Geometry check sheet. Reference: the model listing, model coordinates, mm. Coordinates: 2 decimals unless noted, no trailing zeros. Write each loop counter-clockwise with the first axis right and the second up, starting at its lowest first coordinate (ties: lowest second). Pieces come first, ordered by that corner, then holes. Notation, with made-up numbers: (-38.5, 12) -> (-29.5, 12) arc R10 cw to (-29.5, 18) -> close; hole circle Ø11 at (28.25, 72). An arc over 180 degrees is marked (long way). Answer as CSV lines item,"result".
Autodesk Inventor part; units mm, degrees
ref_plane "YZ Plane" through (0, 0, 0) normal (1, 0, 0) x (0, 1, 0)
ref_plane "XZ Plane" through (0, 0, 0) normal (0, 1, 0) x (-1, 0, 0)
ref_plane "XY Plane" through (0, 0, 0) normal (0, 0, 1) x (1, 0, 0)
sketch "스케치1" plane through (0, 0, 0) normal (0, 1, 0) x (-1, 0, 0)
  line L0 (195, 76.5) -> (-195, 76.5)
  line L1 (-195, 76.5) -> (-195, -76.5)
  line L2 (-195, -76.5) -> (195, -76.5)
  line L3 (195, -76.5) -> (195, 76.5)
  line L4 (195, 76.5) -> (-195, -76.5) construction
  line L5 (-195, 76.5) -> (195, -76.5) construction
  point P0 (0, 0)
  dimension "d0" = 390
  dimension "d1" = 153
extrude "돌출1" add sketch "스케치1" along normal blind 3
sketch "스케치2" plane through (0, 3, 0) normal (0, 1, 0) x (1, 0, 0)
  line L0 (-101, -167.7961) -> (-101, 220.4195)
  line L1 (-195, 76.5) -> (-195, -76.5)
  line L2 (-195, -76.5) -> (195, -76.5)
  circle A0 centre (-101, -31.5) radius 2
  circle A1 centre (-101, 33.5) radius 2
  line L3 (195, -76.5) -> (195, 76.5)
  line L4 (-91, -255.1075) -> (-91, 213.2428)
  line L5 (-111, -276.0921) -> (-111, 192.2583)
  line L6 (-190, -202.8267) -> (-190, 265.5236)
  line L7 (190, -180.3404) -> (190, 288.01)
  line L8 (-211.2868, -71.5) -> (199.2371, -71.5)
  circle A2 centre (12.5, -49.5) radius 2
  circle A3 centre (77.5, -49.5) radius 2
  circle A4 centre (12.5, 49.5) radius 2
  circle A5 centre (77.5, 49.5) radius 2
  line L9 (12.5, -49.5) -> (99.2818, -49.5) construction
  line L10 (12.5, 49.5) -> (77.5, 49.5) construction
  line L11 (195, 76.5) -> (-195, 76.5)
  dimension "d4" = 94
  dimension "d10" = 4
  dimension "d11" = 4
  dimension "d23" = 10
  dimension "d24" = 10
  dimension "d25" = 5
  dimension "d26" = 5
  dimension "d27" = 5
  dimension "d38" = 4
  dimension "d39" = 4
  dimension "d40" = 4
  dimension "d41" = 4
  dimension "d42" = 65
  dimension "d43" = 65
  dimension "d44" = 117.5
  dimension "d45" = 117.5
  dimension "d46" = 27
  dimension "d47" = 27
extrude "돌출2" cut sketch "스케치2" against normal up to surface (3 mm away) contours A0 L0 | L0 A0 | A1 L0 | L0 A1 | A2 | A3 | A4 | A5
sketch "스케치3" plane through (0, 0, 0) normal (0, -1, 0) x (1, 0, 0)
  line L0 (-35, 25) -> (170, 25)
  line L1 (170, 25) -> (170, -20)
  line L2 (170, -20) -> (-35, -20)
  line L3 (-35, -20) -> (-35, 25)
  line L4 (-35, 25) -> (170, -20) construction
  line L5 (170, 25) -> (-35, -20) construction
  line L6 (195, 76.5) -> (195, -76.5)
  line L7 (-165, 33.5) -> (-145, 33.5)
  line L8 (-145, 33.5) -> (-145, -36.5)
  line L9 (-145, -36.5) -> (-165, -36.5)
  line L10 (-165, -36.5) -> (-165, 33.5)
  line L11 (195, -76.5) -> (-195, -76.5)
  line L12 (-195, -76.5) -> (-195, 76.5)
  point P0 (0, 0)
  point P1 (67.5, 2.5)
  dimension "d28" = 205
  dimension "d29" = 25
  dimension "d30" = 45
  dimension "d31" = 20
  dimension "d34" = 70
  dimension "d35" = 20
  dimension "d36" = 110
  dimension "d37" = 30
extrude "돌출3" cut sketch "스케치3" against normal blind 10
sketch "스케치6" plane through (0, 0, 0) normal (0, -1, 0) x (1, 0, 0)
  line L0 (-184, -66.5) -> (-180, -66.5) construction
  line L1 (-184, -68.5) -> (-180, -68.5)
  line L2 (-180, -64.5) -> (-184, -64.5)
  arc A0 (-184, -64.5) -> (-184, -68.5) centre (-184, -66.5) ccw
  arc A1 (-180, -68.5) -> (-180, -64.5) centre (-180, -66.5) ccw
  line L3 (-195, -76.5) -> (-195, 76.5)
  line L4 (195, -76.5) -> (-195, -76.5)
  line L5 (0, -8.9008) -> (0, 5.7448)
  line L6 (-2.4122, 0) -> (4.9846, 0)
  line L7 (184, -66.5) -> (180, -66.5) construction
  line L8 (184, -68.5) -> (180, -68.5)
  line L9 (180, -64.5) -> (184, -64.5)
  arc A2 (184, -68.5) -> (184, -64.5) centre (184, -66.5) ccw
  arc A3 (180, -64.5) -> (180, -68.5) centre (180, -66.5) ccw
  line L10 (-184, 66.5) -> (-180, 66.5) construction
  line L11 (-184, 68.5) -> (-180, 68.5)
  line L12 (-180, 64.5) -> (-184, 64.5)
  arc A4 (-184, 68.5) -> (-184, 64.5) centre (-184, 66.5) ccw
  arc A5 (-180, 64.5) -> (-180, 68.5) centre (-180, 66.5) ccw
  line L13 (184, 66.5) -> (180, 66.5) construction
  line L14 (184, 68.5) -> (180, 68.5)
  line L15 (180, 64.5) -> (184, 64.5)
  arc A6 (184, 64.5) -> (184, 68.5) centre (184, 66.5) ccw
  arc A7 (180, 68.5) -> (180, 64.5) centre (180, 66.5) ccw
  point P0 (0, 0)
  point P1 (-182, -66.5)
  point P2 (182, -66.5)
  point P3 (-182, 66.5)
  point P4 (182, 66.5)
  dimension "d87" = 4
  dimension "d88" = 4
  dimension "d89" = 13
  dimension "d90" = 10
extrude "돌출5" cut sketch "스케치6" against normal blind 10
equation "\"d45\" = d44"
equation "\"d47\" = d46"
properties part number "발 받침대 받침_윗면"
Item 1: Cross-section at A-A, the plane z = 13. Record the cut outline in (x, y), plus the area to 3 significant figures.
Responses:
outline,"(-195, 0) -> (-165, 0) -> (-165, 3) -> (-195, 3) -> close; (-145, 0) -> (-35, 0) -> (-35, 3) -> (-145, 3) -> close; (170, 0) -> (195, 0) -> (195, 3) -> (170, 3) -> close"
area,"495 mm2"
Item 2: Cross-section at B-B, the plane x = 125.5. Record the cut outline in (y, z), plus the area to 3 significant figures.
Responses:
outline,"(0, -76.5) -> (3, -76.5) -> (3, -20) -> (0, -20) -> close; (0, 25) -> (3, 25) -> (3, 76.5) -> (0, 76.5) -> close"
area,"324 mm2"
Item 3: Depth check by flat-ended pin: pin 1 Ø3 at (x, z) = (-101, -33.5) entering from +Y. Enter the tip coordinate at first touch or a pass-through.
Responses:
pin 1,"passes through"
Item 4: Cross-section at C-C, the plane y = 0.9. Count the separate pieces of the cut face and the enclosed holes in it, plus the area to 3 significant figures.
Responses:
separate pieces,"1"
enclosed holes,"12"
area,"48,900 mm2"
Item 5: Thickness scan on probe 1 along Z at (x, y) = (12.5, 1.3); probe 2 along X at (y, z) = (2.65, 14); probe 3 along Z at (x, y) = (-101, 1.1). Record the ranges inside material, lowest first.
Responses:
probe 1,"z = -76.5 to -51.5, -47.5 to -20, 25 to 47.5, 51.5 to 76.5"
probe 2,"x = -195 to -165, -145 to -35, 170 to 195"
probe 3,"z = -76.5 to -35.5, -31.5 to 29.5, 33.5 to 76.5"
